Verification items for the finished model (mm, model axes). A direction names the side the tool comes from. Round coordinates to 2 decimals unless told otherwise and drop trailing zeros. Order: outer loops, then holes, each group sorted by start corner. A loop starts at its lowest first (then second) coordinate and runs counter-clockwise, first axis right, second up. Notation, with made-up numbers: M 44,-20 L 77,-20 A12 ccw 77,-2 Z; hole C 6.25,51 d5. An arc over 180 degrees is marked long. Write item = value, one per line. Start each with the question number.
from build123d import *

# Parameters (mm, degrees)
EXTRUDE_1_DEPTH = 4
SKETCH_2_W      = 132
SKETCH_2_H      = 5.543167705
EXTRUDE_2_DEPTH = 5


with BuildPart() as part:
    # 스케치1 → 보스-돌출1 (new body)
    with BuildSketch(Plane.XY):
        with BuildLine():
            Line((100, 0), (-100, 0))
            Line((-100, 0), (-100, 40))
            Line((-100, 40), (-74, 40))
            Line((-74, 40), (-74, 20))
            ThreePointArc((-74, 20), (-70, 16), (-66, 20))
            Line((-66, 20), (-66, 40))
            Line((-66, 40), (66, 40))
            Line((66, 40), (66, 20))
            ThreePointArc((66, 20), (70, 16), (74, 20))
            Line((74, 20), (74, 40))
            Line((74, 40), (100, 40))
            Line((100, 40), (100, 0))
        make_face()
    extrude(amount=EXTRUDE_1_DEPTH)

    # 스케치2 → 보스-돌출2 (add)
    with BuildSketch(Plane.XY.offset(4)):
        with BuildLine():
            Line((-74, 34.456832295), (-74, 40))
            Line((-74, 40), (-100, 40))
            Line((-100, 40), (-100, 0))
            Line((-100, 0), (-85, 0))
            Line((-85, 0), (-85, 20))
            ThreePointArc((-85, 20), (-81.937336386, 29.082951062), (-74, 34.456832295))
        make_face()
        with Locations((0, 37.228416147)):
            Rectangle(SKETCH_2_W, SKETCH_2_H)
        with BuildLine():
            Line((74, 40), (74, 34.456832295))
            ThreePointArc((74, 34.456832295), (81.937336386, 29.082951062), (85, 20))
            Line((85, 20), (85, 0))
            Line((85, 0), (100, 0))
            Line((100, 0), (100, 40))
            Line((100, 40), (74, 40))
        make_face()
    extrude(amount=EXTRUDE_2_DEPTH)


solid = part.part
1) Cross-section at C-C, the plane x = 57.5. Enter the section's corners in (y, z).
2) Cross-section at D-D, the plane y = 18. Enter the section's corners in (x, z), then the cut area to 3 significant figures.
3) Release check for a two-part mould opening along X. For faces 1 (the flat face through (100, 20, 4)), 2 (the flat face through (1, 20, 0)), 3 (the flat face through (74, 32, 2)) record: pulls with the +X half, pulls with the -X half, needs draft (parallel to the pull), parting line crosses it, or undercut.
4) Access from +Z, -Z, +X, -X, +Y, -Y to the whole of each face (thin tool, end or side, straight path). Record for faces 4 (the cylindrical face through (-82, 29, 6)), 5 (the flat face through (-66, 32, 2)), 6 (the flat face through (87, 40, 4)).
5) Cross-section at A-A, the plane y = 37. Enter the section's corners in (x, z), then the cut area to 3 significant figures.
6) Cross-section at B-B, the plane z = 6.25. Enter the section's corners in (x, y), then the cut area to 3 significant figures.
7) Scan lines: probe 1 along X at (y, z) = (36.5, 2.5); probe 2 along X at (y, z) = (17.5, 6.5); probe 3 along Z at (x, y) = (34, 7.5). Record each from-to range of solid material in increasing order.
8) Gauge pin test, flat ends, axial feed: P1, Ø10.5, axis at x = -42, y = 10, coming from the +Z side; P2, Ø1, axis at x = -56, z = 6, coming from the -Y side; P3, Ø12, axis at x = 72, y = 8.5, coming from the -Z side. Record the tip position at first contact, or that the pin passes through.
Geometry results:
q1.outline = M 0,0 L 40,0 L 40,9 L 34.46,9 L 34.46,4 L 0,4 Z
q2.outline = M -100,0 L -73.46,0 L -73.46,4 L -85,4 L -85,9 L -100,9 Z; M -66.54,0 L 66.54,0 L 66.54,4 L -66.54,4 Z; M 73.46,0 L 100,0 L 100,9 L 85,9 L 85,4 L 73.46,4 Z
q2.area = 895 mm^2
q3.face_1 = pulls with the +X half
q3.face_2 = needs draft
q3.face_3 = undercut
q4.face_4 = +Z, -Y
q4.face_5 = +Z, -Z, +Y
q4.face_6 = +Z, -Z, +X, -X, +Y
q5.outline = M -100,0 L -74,0 L -74,9 L -100,9 Z; M -66,0 L 66,0 L 66,9 L -66,9 Z; M 74,0 L 100,0 L 100,9 L 74,9 Z
q5.area = 1,660 mm^2
q6.outline = M -100,0 L -85,0 L -85,20 A15 cw -74,34.46 L -74,40 L -100,40 Z; M -66,34.46 L 66,34.46 L 66,40 L -66,40 Z; M 74,34.46 A15 cw 85,20 L 85,0 L 100,0 L 100,40 L 74,40 Z
q6.area = 2,140 mm^2
q7.probe_1 = -100 to -74, -66 to 66, 74 to 100
q7.probe_2 = -100 to -85, 85 to 100
q7.probe_3 = 0 to 4
q8.P1 = 4
q8.P2 = 34.46
q8.P3 = 0
